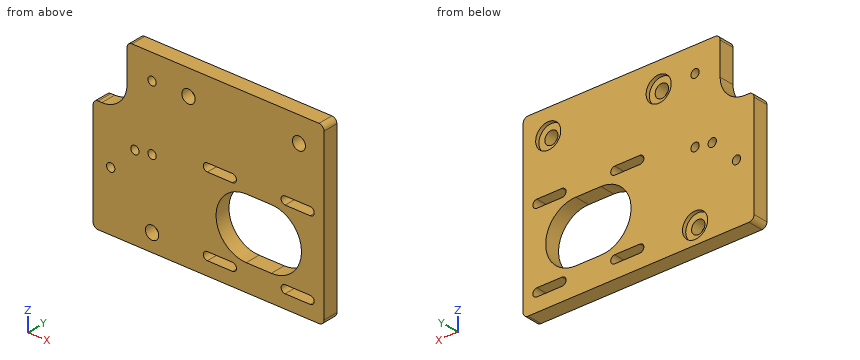
```python
from build123d import *

# Parameters (mm, degrees)
SKETCH3_R                   = 2.6
BOSS_EXTRUDE1_DEPTH         = 6
FILLET1_R                   = 10
M3_CLEARANCE_HOLE1_D        = 3.2
M4X0_7_TAPPED_HOLE1_D       = 3.3
FILLET2_R                   = 2
SKETCH5_R                   = 5
COUNTERBORE_DEPTH           = 1.5
SKETCH14_R                  = 5
SKETCH14_R_2                = 1.6
HOLE_FILLER_DEPTH           = 6
M5_HOLE_RELOCATION_OPTION_R = 5
CUT_EXTRUDE1_DEPTH          = 1.5
M5_CLEARANCE_HOLE1_D        = 5.3
M4X0_7_TAPPED_HOLE2_D       = 3.3


with BuildPart() as part:
    # Sketch3 → Boss-Extrude1 (new body)
    with BuildSketch(Plane(origin=(0, 0, 0), x_dir=(1, 0, 0), z_dir=(0, 1, 0))):
        Polygon((0, 0), (78.5, 0), (78.5, 70), (0, 70), (-13.5, 70), (-13.5, 25), (0, 25), align=None)
        with Locations(Location((10, 56, 0), (0, 0, 270))):
            Circle(SKETCH3_R, mode=Mode.SUBTRACT)
        with Locations(Location((10, 10, 0), (0, 0, 270))):
            Circle(SKETCH3_R, mode=Mode.SUBTRACT)
        with Locations(Location((68.5, 10, 0), (0, 0, 270))):
            Circle(SKETCH3_R, mode=Mode.SUBTRACT)
        with Locations(Location((30, 10, 0), (0, 0, 270))):
            Circle(SKETCH3_R, mode=Mode.SUBTRACT)
        with BuildLine():
            Line((47.5, 59.5), (57.5, 59.5))
            ThreePointArc((57.5, 59.5), (69.5, 47.5), (57.5, 35.5))
            Line((57.5, 35.5), (47.5, 35.5))
            ThreePointArc((47.5, 35.5), (35.5, 47.5), (47.5, 59.5))
        make_face(mode=Mode.SUBTRACT)
        with BuildLine():
            Line((32, 64.6), (42, 64.6))
            ThreePointArc((42, 64.6), (43.6, 63), (42, 61.4))
            Line((42, 61.4), (32, 61.4))
            ThreePointArc((32, 61.4), (30.4, 63), (32, 64.6))
        make_face(mode=Mode.SUBTRACT)
        with BuildLine():
            Line((63, 64.6), (73, 64.6))
            ThreePointArc((73, 64.6), (74.6, 63), (73, 61.4))
            Line((73, 61.4), (63, 61.4))
            ThreePointArc((63, 61.4), (61.4, 63), (63, 64.6))
        make_face(mode=Mode.SUBTRACT)
        with BuildLine():
            Line((63, 33.6), (73, 33.6))
            ThreePointArc((73, 33.6), (74.6, 32), (73, 30.4))
            Line((73, 30.4), (63, 30.4))
            ThreePointArc((63, 30.4), (61.4, 32), (63, 33.6))
        make_face(mode=Mode.SUBTRACT)
        with BuildLine():
            Line((32, 33.6), (42, 33.6))
            ThreePointArc((42, 33.6), (43.6, 32), (42, 30.4))
            Line((42, 30.4), (32, 30.4))
            ThreePointArc((32, 30.4), (30.4, 32), (32, 33.6))
        make_face(mode=Mode.SUBTRACT)
    extrude(amount=BOSS_EXTRUDE1_DEPTH)

    # Fillet1
    fillet1_edges = [part.edges().sort_by_distance(p)[0] for p in [
        (0, 3, -25),
    ]]
    fillet(fillet1_edges, radius=FILLET1_R)

    # M3 Clearance Hole1 (through all)
    with Locations(Plane(origin=(0, 6, 0), x_dir=(1, 0, 0), z_dir=(0, 1, 0))):
        with Locations((10, 64.325), (-6.5, 64.325)):
            Hole(M3_CLEARANCE_HOLE1_D / 2)

    # M4x0.7 Tapped Hole1 (through all)
    with Locations(Plane(origin=(0, 6, 0), x_dir=(1, 0, 0), z_dir=(0, 1, 0))):
        with Locations((-6.5, 46.325), (10, 35.7)):
            Hole(M4X0_7_TAPPED_HOLE1_D / 2)

    # Fillet2
    fillet2_edges = [part.edges().sort_by_distance(p)[0] for p in [
        (-13.5, 3, -25),
        (-13.5, 3, -70),
        (78.5, 3, -70),
        (78.5, 3, 0),
        (0, 3, 0),
    ]]
    fillet(fillet2_edges, radius=FILLET2_R)

    # Sketch5 → Counterbore (cut)
    with BuildSketch(Plane(origin=(0, 6, 0), x_dir=(1, 0, 0), z_dir=(0, 1, 0))):
        with Locations(Location((10, 56, 0), (0, 0, 270))):
            Circle(SKETCH5_R)
        with Locations(Location((10, 10, 0), (0, 0, 270))):
            Circle(SKETCH5_R)
        with Locations(Location((30, 10, 0), (0, 0, 270))):
            Circle(SKETCH5_R)
        with Locations(Location((68.5, 10, 0), (0, 0, 270))):
            Circle(SKETCH5_R)
    extrude(amount=-COUNTERBORE_DEPTH, mode=Mode.SUBTRACT)

    # Sketch14 → Hole Filler (add)
    with BuildSketch(Plane(origin=(0, 6, 0), x_dir=(1, 0, 0), z_dir=(0, 1, 0))):
        with Locations((10, 10)):
            Circle(SKETCH14_R)
        with Locations((10, 56)):
            Circle(SKETCH14_R)
        with Locations((-6.5, 64.325)):
            Circle(SKETCH14_R_2)
        with Locations((10, 64.325)):
            Circle(SKETCH14_R_2)
        with Locations((30, 10)):
            Circle(SKETCH14_R)
    extrude(amount=-HOLE_FILLER_DEPTH)

    # M5 hole relocation option → Cut-Extrude1 (cut)
    with BuildSketch(Plane(origin=(0, 6, 0), x_dir=(1, 0, 0), z_dir=(0, 1, 0))):
        with Locations(Location((24.5, 10, 0), (0, 0, 270))):
            Circle(M5_HOLE_RELOCATION_OPTION_R)
        with Locations(Location((10, 63, 0), (0, 0, 270))):
            Circle(M5_HOLE_RELOCATION_OPTION_R)
    extrude(amount=-CUT_EXTRUDE1_DEPTH, mode=Mode.SUBTRACT)

    # M5 Clearance Hole1 (through all)
    with Locations(Plane(origin=(0, 4.5, 0), x_dir=(1, 0, 0), z_dir=(0, 1, 0))):
        with Locations((24.5, 10), (10, 63)):
            Hole(M5_CLEARANCE_HOLE1_D / 2)

    # M4x0.7 Tapped Hole2 (through all)
    with Locations(Plane(origin=(0, 6, 0), x_dir=(1, 0, 0), z_dir=(0, 1, 0))):
        with Locations((10, 10), (3.145, 36.68)):
            Hole(M4X0_7_TAPPED_HOLE2_D / 2)


solid = part.part
```
The listing builds one solid part. Answer for the finished solid, in the listing's coordinates (mm). Round coordinates to 2 decimals unless told otherwise and drop trailing zeros. Write each loop counter-clockwise with the first axis right and the second up, starting at its lowest first coordinate (ties: lowest second). Pieces come first, ordered by that corner, then holes. Notation, with made-up numbers: (41, 13) -> (84, 13) arc R8 ccw to (84, 18) -> close; hole circle Ø9 at (-24, -15.75). An arc over 180 degrees is marked (long way). Use CSV: the item, a comma, the result in double quotes. Start each with the question number.
(1) Section B-B on z = -10 is taken. Give the vertices of the cut face in (x, y).
(2) Consider L1, parallel to X at y = 3.1, z = -10; L2, parallel to Z at x = 70.5, y = 4.1; L3, parallel to X at y = 3.65, z = -8.5. Determine where each line is inside the solid, lowest interval first. Write a range as from..to.
(3) Each of these flat-tipped pins is pushed along its axis until it touches: pin 1 (9 mm diameter, centred on x = 68.5, z = -10, fed in from +Y); pin 2 (0.8 mm diameter, centred on x = -10.5, y = 3, fed in from +Z). Where does it stop, or does it pass through?
(4) Section C-C on x = 68.5 is taken. Give the vertices of the cut face in (y, z).
(5) Section D-D on z = -23 is taken. Give the vertices of the cut face in (x, y), then the cut area to 3 significant figures.
(6) Section A-A on x = 24.5 is taken. Give the vertices of the cut face in (y, z), then the cut area to 3 significant figures.
A:
1,outline,"(0, 0) -> (8.35, 0) -> (8.35, 6) -> (0, 6) -> close; (11.65, 0) -> (21.85, 0) -> (21.85, 4.5) -> (19.5, 4.5) -> (19.5, 6) -> (11.65, 6) -> close; (27.15, 0) -> (65.9, 0) -> (65.9, 4.5) -> (63.5, 4.5) -> (63.5, 6) -> (29.5, 6) -> (29.5, 4.5) -> (27.15, 4.5) -> close; (71.1, 0) -> (78.5, 0) -> (78.5, 6) -> (73.5, 6) -> (73.5, 4.5) -> (71.1, 4.5) -> close"
2,L1,"x = 0..8.35, 11.65..21.85, 27.15..65.9, 71.1..78.5"
2,L2,"z = -70..-64.6, -61.4..-33.6, -30.4..-11.66, -8.34..0"
2,L3,"x = 0..9.31, 10.69..22.32, 26.68..66.38, 70.62..78.5"
3,pin 1,"stops at y = 4.5"
3,pin 2,"stops at z = -25"
4,outline,"(0, -70) -> (6, -70) -> (6, -64.6) -> (0, -64.6) -> close; (0, -61.4) -> (6, -61.4) -> (6, -52.3) -> (0, -52.3) -> close; (0, -42.7) -> (6, -42.7) -> (6, -33.6) -> (0, -33.6) -> close; (0, -30.4) -> (6, -30.4) -> (6, -15) -> (4.5, -15) -> (4.5, -12.6) -> (0, -12.6) -> close; (0, -7.4) -> (4.5, -7.4) -> (4.5, -5) -> (6, -5) -> (6, 0) -> (0, 0) -> close"
5,outline,"(-4, 0) -> (78.5, 0) -> (78.5, 6) -> (-4, 6) -> close"
5,area,"495 mm²"
6,outline,"(0, -70) -> (6, -70) -> (6, -15) -> (4.5, -15) -> (4.5, -12.65) -> (0, -12.65) -> close; (0, -7.35) -> (4.5, -7.35) -> (4.5, -5) -> (6, -5) -> (6, 0) -> (0, 0) -> close"
6,area,"381 mm²"
